from build123d import *

# Parameters (mm, degrees)
SKETCH1_W           = 114.3
SKETCH1_H           = 38.1
BOSS_EXTRUDE1_DEPTH = 6.35
SKETCH2_R           = 11.1125
CUT_EXTRUDE1_DEPTH  = 61.57513929
SKETCH3_W           = 66.543997706
SKETCH3_H           = 12.7
CUT_EXTRUDE2_DEPTH  = 61.57513929


with BuildPart() as part:
    # Sketch1 → Boss-Extrude1 (new body)
    with BuildSketch(Plane.XY):
        Rectangle(SKETCH1_W, SKETCH1_H)
    extrude(amount=BOSS_EXTRUDE1_DEPTH)

    # Sketch2 → Cut-Extrude1 (cut, through all)
    with BuildSketch(Plane.XY.offset(6.35)):
        with Locations((-38.205321874, 0)):
            Circle(SKETCH2_R)
        with Locations((38.1, 0)):
            Circle(SKETCH2_R)
    extrude(amount=-CUT_EXTRUDE1_DEPTH, mode=Mode.SUBTRACT)

    # Sketch3 → Cut-Extrude2 (cut, through all)
    with BuildSketch(Plane.XY.offset(6.35)):
        Rectangle(SKETCH3_W, SKETCH3_H)
    extrude(amount=-CUT_EXTRUDE2_DEPTH, mode=Mode.SUBTRACT)


solid = part.part
Check sheet for the modelled part. Datum: model origin and axes. Units: mm. A direction names the side the tool comes from. Give positions to 0.01 mm unless a question says otherwise; leave off trailing zeros. Write each loop counter-clockwise with the first axis right and the second up, starting at its lowest first coordinate (ties: lowest second). Pieces come first, ordered by that corner, then holes. Notation, with made-up numbers: (57.25, 42.5) -> (112.25, 42.5) arc R11 cw to (112.25, 61.5) -> close; hole circle Ø2 at (61.5, 8). An arc over 180 degrees is marked (long way). One line per item, written item: value. Start each with the question number.
Item 1: Draft check along Y on faces 1 (the cylindrical face through (49.206, -0.394, 3.219)), 2 (the flat face through (-1, 19.05, 3)), 3 (the flat face through (0, 6.35, 3)), 4 (the flat face through (-57.15, 0, 3)). Enter one of: +Y half, -Y half, draft (parallel to the pull), parting line (faces both ways), or undercut.
Item 2: Material ranges on probe 1 along X at (y, z) = (0, 2.75); probe 2 along Y at (x, z) = (-17.5, 5.75); probe 3 along Y at (x, z) = (38.1, 2), recorded low to high. Write a range as from..to.
Item 3: Tool access check on faces 5 (the flat face through (0, -6.35, 3)), 6 (the flat face through (57.15, 0, 3)). Record the directions out of +Z, -Z, +X, -X, +Y, -Y that give a thin tool (end or side, any length) a straight path to the whole face; none if there is none.
Item 4: Gauge pin test, flat end, axial feed: pin 1 (18 mm diameter, centred on x = -38.21, y = 0, fed in from +Z). Record the tip position at first contact, or that the pin passes through.
Item 5: Section check C-C on x = 6. Record the cut outline in (y, z).
Item 6: Section check D-D on y = 8. Record the cut outline in (x, z).
Item 7: Section check B-B on y = 0. Record the cut outline in (x, z).
Results list:
1. face 1: undercut
1. face 2: +Y half
1. face 3: undercut
1. face 4: draft
2. probe 1: -57.15..-49.32, 49.21..57.15
2. probe 2: -19.05..-6.35, 6.35..19.05
2. probe 3: -19.05..-11.11, 11.11..19.05
3. face 5: +Z, -Z
3. face 6: +Z, -Z, +X, +Y, -Y
4. pin 1: through
5. outline: (-19.05, 0) -> (-6.35, 0) -> (-6.35, 6.35) -> (-19.05, 6.35) -> close; (6.35, 0) -> (19.05, 0) -> (19.05, 6.35) -> (6.35, 6.35) -> close
6. outline: (-57.15, 0) -> (-45.92, 0) -> (-45.92, 6.35) -> (-57.15, 6.35) -> close; (-30.49, 0) -> (30.39, 0) -> (30.39, 6.35) -> (-30.49, 6.35) -> close; (45.81, 0) -> (57.15, 0) -> (57.15, 6.35) -> (45.81, 6.35) -> close
7. outline: (-57.15, 0) -> (-49.32, 0) -> (-49.32, 6.35) -> (-57.15, 6.35) -> close; (49.21, 0) -> (57.15, 0) -> (57.15, 6.35) -> (49.21, 6.35) -> close
